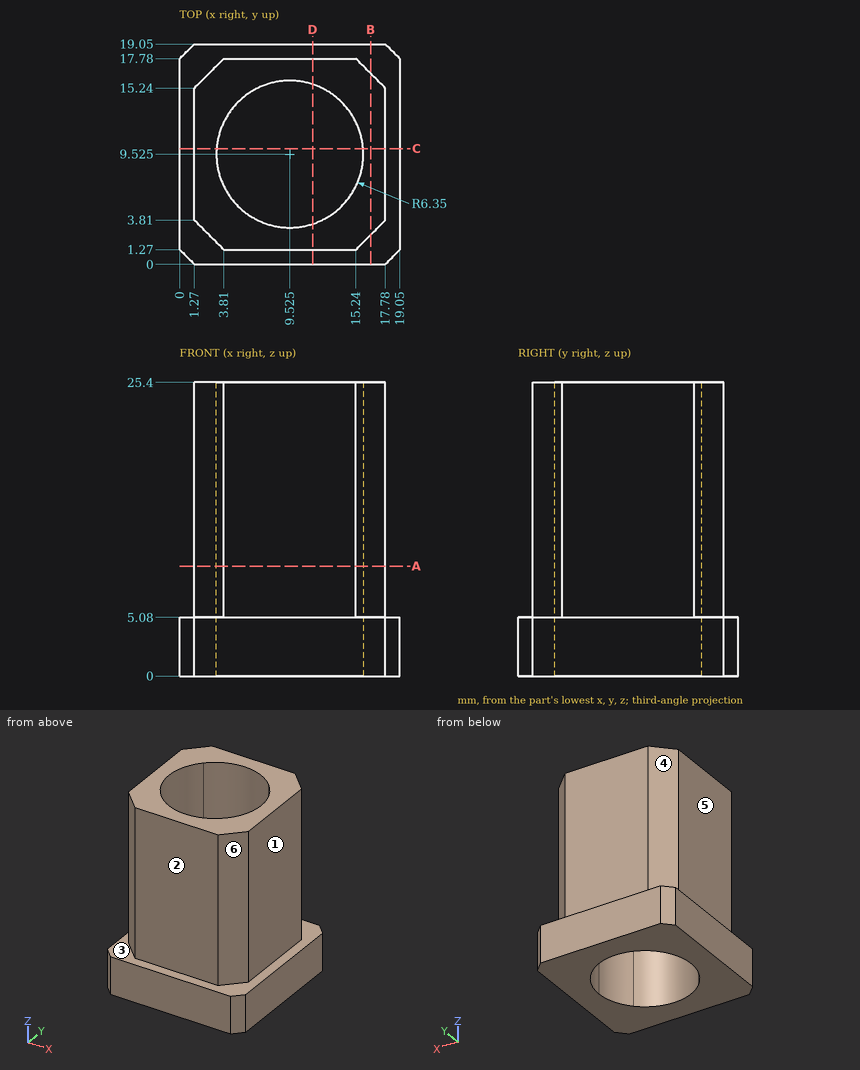
Part print with two shaded views. Sizes in mm from the minimum x, y, z corner. A direction names the side the tool comes from. Give positions to 0.01 mm unless a question says otherwise; leave off trailing zeros. Order: outer loops, then holes, each group sorted by start corner. A loop starts at its lowest first (then second) coordinate and runs counter-clockwise, first axis right, second up.
1) Saw through at A-A, the plane z = 9.5. Write the cut outline in (x, y) (3 decimals).
2) Mould opens along Y. For the marked faces 4, 5 and 6 say: +Y half, -Y half, draft (parallel to the pull), parting line (faces both ways), or undercut.
3) Saw through at B-B, the plane x = 16.5. Write the cut outline in (y, z).
4) Saw through at D-D, the plane x = 11.5. Write the cut outline in (y, z).
5) Saw through at C-C, the plane y = 10. Write the cut outline in (x, z).
6) 3-axis set-ups, long thin cutter, end or side, ignore diameter. For the marked faces 1, 2 and 3: which of +Z, -Z, +X, -X, +Y, -Y reach the whole face in a straight line?
7) Wall check: probe 1 along X at (y, z) = (9.5, 21.75); probe 2 along Y at (x, z) = (4, 1.75) (3 decimals); probe 3 along Y at (x, z) = (4.5, 1.5). Give the ranges that are in metal, low to high.
8) Pin check, flat tips, straight feed: pin 1 (6 mm diameter, centred on x = 16.5, z = 15.5, fed in from -Y); pin 2 (5.5 mm diameter, centred on x = 11.5, z = 17, fed in from +Y); pin 3 (9 mm diameter, centred on y = 11.5, z = 11, fed in from +X); pin 4 (3 mm diameter, centred on x = 15.5, z = 6, fed in from -Y). Stop position of each tip, or through.
Computed:
1. outline: (1.27, 3.81) - (3.81, 1.27) - (15.24, 1.27) - (17.78, 3.81) - (17.78, 15.24) - (15.24, 17.78) - (3.81, 17.78) - (1.27, 15.24) - close; hole circle Ø12.7 at (9.525, 9.525)
2. face 4: +Y half
2. face 5: draft
2. face 6: -Y half
3. outline: (0, 0) - (19.05, 0) - (19.05, 5.08) - (16.52, 5.08) - (16.52, 25.4) - (2.53, 25.4) - (2.53, 5.08) - (0, 5.08) - close
4. outline: (0, 0) - (3.49, 0) - (3.49, 25.4) - (1.27, 25.4) - (1.27, 5.08) - (0, 5.08) - close; (15.56, 0) - (19.05, 0) - (19.05, 5.08) - (17.78, 5.08) - (17.78, 25.4) - (15.56, 25.4) - close
5. outline: (0, 0) - (3.19, 0) - (3.19, 25.4) - (1.27, 25.4) - (1.27, 5.08) - (0, 5.08) - close; (15.86, 0) - (19.05, 0) - (19.05, 5.08) - (17.78, 5.08) - (17.78, 25.4) - (15.86, 25.4) - close
6. face 1: +Z, +X, +Y, -Y
6. face 2: +Z, +X, -X, -Y
6. face 3: +Z
7. probe 1: x = 1.27 to 3.18, 15.87 to 17.78
7. probe 2: y = 0 to 6.395, 12.655 to 19.05
7. probe 3: y = 0 to 5.64, 13.41 to 19.05
8. pin 1: stops at y = 1.27
8. pin 2: stops at y = 17.78
8. pin 3: stops at x = 17.78
8. pin 4: stops at y = 0
